Autodesk Inventor part; units mm, degrees
ref_plane "YZ Plane" through (0, 0, 0) normal (1, 0, 0) x (0, 1, 0)
ref_plane "XZ Plane" through (0, 0, 0) normal (0, 1, 0) x (-1, 0, 0)
ref_plane "XY Plane" through (0, 0, 0) normal (0, 0, 1) x (1, 0, 0)
sketch "Sketch1" plane through (0, 0, 0) normal (1, 0, 0) x (0, 1, 0)
  line L0 (0, 0) -> (-20, 0)
  line L1 (-20, 0) -> (-20, -2)
  line L2 (-20, -2) -> (0, -2)
  line L3 (0, -2) -> (0, 0)
  line L4 (0, 0) -> (-2, 0)
  line L5 (-2, 0) -> (-2, -20)
  line L6 (-2, -20) -> (0, -20)
  line L7 (0, -20) -> (0, 0)
  dimension "d0" = 20
  dimension "d1" = 2
  dimension "d2" = 2
  dimension "d3" = 20
extrude "Extrusion1" add sketch "Sketch1" along normal blind 120
sketch "Sketch2" plane through (0, 0, 0) normal (0, 1, 0) x (1, 0, 0)
  line L0 (0, 20) -> (0, 0)
  line L1 (0, 0) -> (0, 10)
  line L2 (0, 10) -> (30, 10)
  circle A0 centre (30, 10) radius 2.5
  dimension "d6" = 10
  dimension "d7" = 30
  dimension "d8" = 5
extrude "Extrusion2" cut sketch "Sketch2" against normal blind 120
pattern_linear "Rectangular Pattern1" count 3 spacing 30 along (1, 0, 0) of "Extrusion2"
sketch "Sketch3" plane through (0, -20, 0) normal (0, 0, 1) x (1, 0, 0)
  line L0 (0, 0) -> (0, 18)
  line L1 (0, 0) -> (0, 10)
  line L2 (0, 10) -> (30, 10)
  circle A0 centre (30, 10) radius 2.5
  point P0 (0, 20)
  dimension "d14" = 10
  dimension "d15" = 30
  dimension "d16" = 5
extrude "Extrusion3" cut sketch "Sketch3" against normal blind 120
pattern_linear "Rectangular Pattern2" count 3 spacing 30 along (1, 0, 0) of "Extrusion3"
sketch "Sketch4" plane through (0, -2, -20) normal (0, -1, 0) x (1, 0, 0)
  line L0 (0, 0) -> (120, 0)
  line L1 (21.4627, 0) -> (41.4627, 0)
  line L2 (41.4627, 0) -> (41.4627, 2)
  line L3 (41.4627, 2) -> (21.4627, 2)
  line L4 (21.4627, 2) -> (21.4627, 0)
  line L5 (21.4627, 0) -> (23.4627, 0)
  line L6 (23.4627, 0) -> (23.4627, 20)
  line L7 (23.4627, 20) -> (21.4627, 20)
  line L8 (21.4627, 20) -> (21.4627, 0)
  point P0 (0, 20)
  dimension "d22" = 20
  dimension "d23" = 2
  dimension "d24" = 2
extrude "Extrusion4" add sketch "Sketch4" along normal blind 120
sketch "Sketch5" plane through (23.4627, -2, -2) normal (1, 0, 0) x (0, 0, -1)
  line L0 (0, -18) -> (0, 0)
  line L1 (-2, -18) -> (0, -18)
  line L2 (-2, -18) -> (-2, -120)
  line L3 (16, -120) -> (-2, -120)
  line L4 (16, -120) -> (16, 0)
  line L5 (0, 0) -> (16, 0)
  line L6 (-2, 2) -> (-2, -18)
  line L7 (-2, -18) -> (0, -18)
  line L8 (0, -18) -> (0, 0)
  line L9 (0, 0) -> (18, 0)
  line L10 (18, 0) -> (18, 2)
  line L11 (18, 2) -> (-2, 2)
  line L12 (18, 2) -> (-2, 2)
  line L13 (-2, 2) -> (8, 2)
  line L14 (8, 2) -> (8, -28)
  circle A0 centre (8, -28) radius 2.5
  dimension "d27" = 30
  dimension "d28" = 5
extrude "Extrusion5" cut sketch "Sketch5" against normal blind 120 contours A0
pattern_linear "Rectangular Pattern3" count 3 spacing 30 along (0, -1, 0) of "Extrusion5"
sketch "Sketch6" plane through (120, 0, -20) normal (0, 0, -1) x (-1, 0, 0)
  line L0 (98.5373, -2) -> (98.5373, -122)
  line L1 (98.5373, -2) -> (98.5373, 0)
  line L2 (98.5373, 0) -> (88.5373, 0)
  line L3 (120, 0) -> (0, 0)
  line L4 (88.5373, 0) -> (88.5373, -30)
  circle A0 centre (88.5373, -30) radius 2.5
  dimension "d34" = 10
  dimension "d35" = 30
  dimension "d36" = 5
extrude "Extrusion6" cut sketch "Sketch6" against normal blind 120
pattern_linear "Rectangular Pattern4" count 3 spacing 30 along (0, -1, 0) of "Extrusion6"
fillet "Fillet1" radius 2 2 edges at (21.4627, -11, -2) (21.4627, -2, -11)
fillet "Fillet2" radius 2 2 edges at (23.4627, -2, -10) (23.4627, -11, -2)
properties part number "lol"
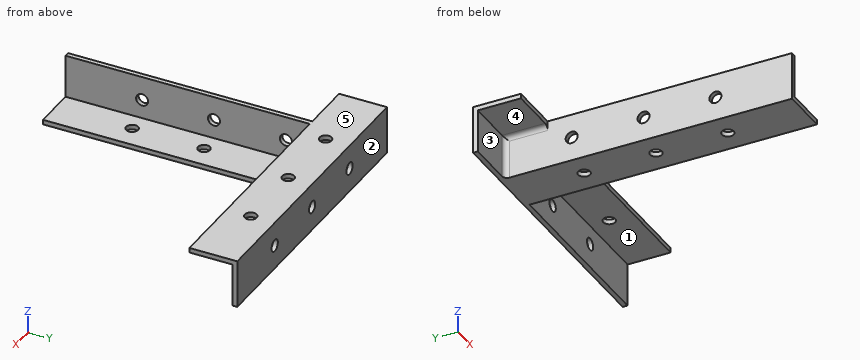
Verification items for the finished model (mm, model axes). Face numbers are marked on the shaded views. A direction names the side the tool comes from. Coordinates: 2 decimals unless noted, no trailing zeros. Loops run counter-clockwise (first coordinate to the right, second up) from the corner with the lowest first, then second, coordinate; pieces in that order, holes last. Notation, with made-up numbers: (16, -10) -> (34, -10) arc R4 cw to (34, -3) -> close; hole circle Ø11 at (73, 8.5). An arc over 180 degrees is marked (long way). Answer in a Markdown table with one row per item.
1) Section check C-C (z = -10). Give the number of separate pieces and of enclosed holes in the cut face, and give its area (3 significant figures).
The answers:
| item | result |
|---|---|
| separate pieces | 7 |
| enclosed holes | 0 |
| area | 422 mm2 |
2) Draft check along Y on the marked faces 1, 2 and 3. Enter one of: released by +Y, released by -Y, zero draft, split by the parting line, or undercut.
The answers:
| item | result |
|---|---|
| face 1 | zero draft |
| face 2 | released by +Y |
| face 3 | released by -Y |
3) Section check A-A (x = 90). Record the cut outline in (y, z), and give its area (3 significant figures).
The answers:
| item | result |
|---|---|
| outline | (-20, -2) -> (-12.5, -2) -> (-12.5, 0) -> (-20, 0) -> close; (-7.5, -2) -> (-2, -2) -> (-2, -7.5) -> (0, -7.5) -> (0, 0) -> (-7.5, 0) -> close; (-2, -20) -> (0, -20) -> (0, -12.5) -> (-2, -12.5) -> close |
| area | 56.0 mm2 |
4) Scan lines: line 1 along Y through (x, z) = (22.35, -10); line 2 along Z through (x, y) = (90, -0.5); line 3 along X through (y, z) = (-103, -17.75). Record each from-to range of solid material in increasing order. Write a range as from..to.
The answers:
| item | result |
|---|---|
| line 1 | y = -122..-92.5, -87.5..-62.5, -57.5..-32.5, -27.5..0 |
| line 2 | z = -20..-12.5, -7.5..0 |
| line 3 | x = 21.46..23.46 |
5) Section check B-B (y = -60). Record the cut outline in (x, z).
The answers:
| item | result |
|---|---|
| outline | (21.46, -20) -> (28.96, -20) -> (28.96, -18) -> (23.46, -18) -> (23.46, -12.5) -> (21.46, -12.5) -> close; (21.46, -7.5) -> (23.46, -7.5) -> (23.46, 0) -> (21.46, 0) -> close; (33.96, -20) -> (41.46, -20) -> (41.46, -18) -> (33.96, -18) -> close |
6) Section check D-D (y = -10). Record the cut outline in (x, z), and give its area (3 significant figures).
The answers:
| item | result |
|---|---|
| outline | (0, -2) -> (19.46, -2) arc R2 cw to (21.46, -4) -> (21.46, -20) -> (41.46, -20) -> (41.46, -18) -> (23.46, -18) -> (23.46, -4) arc R2 cw to (25.46, -2) -> (27.5, -2) -> (27.5, 0) -> (0, 0) -> close; (32.5, -2) -> (57.5, -2) -> (57.5, 0) -> (32.5, 0) -> close; (62.5, -2) -> (87.5, -2) -> (87.5, 0) -> (62.5, 0) -> close; (92.5, -2) -> (120, -2) -> (120, 0) -> (92.5, 0) -> close |
| area | 284 mm2 |
7) Access from +Z, -Z, +X, -X, +Y, -Y to the whole of each face (thin tool, end or side, straight path). Record for the marked faces 4 and 5.
The answers:
| item | result |
|---|---|
| face 4 | -Z, -X, -Y |
| face 5 | +Z, +X, -X, +Y, -Y |
8) Depth check by flat-ended pin: P1, Ø9, axis at x = 28.5, y = -37.5, coming from the +Z side; P2, Ø2, axis at y = -49, z = -18.5, coming from the +X side; P3, Ø9, axis at x = 11, z = -11, coming from the -Y side. Enter the tip coordinate at first touch or a pass-through.
The answers:
| item | result |
|---|---|
| P1 | stops at z = -18 |
| P2 | stops at x = 41.46 |
| P3 | stops at y = -2 |
